```python
from build123d import *

# Parameters (mm, degrees)
SKETCH_1_R          = 15
EXTRUDE_1_DEPTH     = 2
SKETCH_2_R          = 7
EXTRUDE_2_DEPTH     = 10
SKETCH_3_R          = 2
CUT_EXTRUDE_1_DEPTH = 24.452078799
SKETCH_4_R          = 5
CUT_EXTRUDE_2_DEPTH = 25.372115214
CHAMFER_1_SIZE      = 0.2
SKETCH_5_R          = 1.75
CUT_EXTRUDE_3_DEPTH = 10


with BuildPart() as part:
    # 草图1 → 凸台-拉伸1 (new body)
    with BuildSketch(Plane(origin=(0, 0, 0), x_dir=(0, 0, -1), z_dir=(1, 0, 0))):
        Circle(SKETCH_1_R)
    extrude(amount=EXTRUDE_1_DEPTH)

    # 草图2 → 凸台-拉伸2 (add)
    with BuildSketch(Plane(origin=(2, 0, 0), x_dir=(0, 0, -1), z_dir=(1, 0, 0))):
        Circle(SKETCH_2_R)
    extrude(amount=EXTRUDE_2_DEPTH)

    # 草图3 → 切除-拉伸1 (cut, through all)
    with BuildSketch(Plane(origin=(2, 0, 0), x_dir=(0, 0, -1), z_dir=(1, 0, 0))):
        with Locations((0, 11.313708499)):
            Circle(SKETCH_3_R)
        with Locations((8, 8)):
            Circle(SKETCH_3_R)
        with Locations((11.313708499, 0)):
            Circle(SKETCH_3_R)
        with Locations((8, -8)):
            Circle(SKETCH_3_R)
        with Locations((0, -11.313708499)):
            Circle(SKETCH_3_R)
        with Locations((-8, -8)):
            Circle(SKETCH_3_R)
        with Locations((-11.313708499, 0)):
            Circle(SKETCH_3_R)
        with Locations((-8, 8)):
            Circle(SKETCH_3_R)
    extrude(amount=-CUT_EXTRUDE_1_DEPTH, mode=Mode.SUBTRACT)

    # 草图4 → 切除-拉伸2 (cut, through all)
    with BuildSketch(Plane(origin=(12, 0, 0), x_dir=(0, 0, -1), z_dir=(1, 0, 0))):
        Circle(SKETCH_4_R)
    extrude(amount=-CUT_EXTRUDE_2_DEPTH, mode=Mode.SUBTRACT)

    # 倒角1
    chamfer_1_edges = [part.edges().sort_by_distance(p)[0] for p in [
        (0, 0, 15),
        (0, 0, 5),
        (12, 0, 5),
        (2, 0, 15),
        (12, 0, 7),
    ]]
    chamfer(chamfer_1_edges, length=CHAMFER_1_SIZE)

    # 草图5 → 切除-拉伸3 (cut)
    with BuildSketch(Plane(origin=(0, 0, 0), x_dir=(1, 0, 0), z_dir=(0, 1, 0))):
        with Locations(Location((7, 0, 0), (0, 0, 90))):
            Circle(SKETCH_5_R)
    extrude(amount=CUT_EXTRUDE_3_DEPTH, mode=Mode.SUBTRACT)


solid = part.part
```
Model file for the job. Use its own axes, mm. A direction names the side the tool comes from. Coordinates: 2 decimals unless noted, no trailing zeros. Loops run counter-clockwise (first coordinate to the right, second up) from the corner with the lowest first, then second, coordinate; pieces in that order, holes last. Notation, with made-up numbers: (86, 14) -> (101, 14) arc R21 ccw to (101, 31) -> close; hole circle Ø7 at (-4.75, 50.25). An arc over 180 degrees is marked (long way). Answer as a JSON object with one key per item and string values.
Q1. Cut at C-C (x = 10.25). List the corners of the cut face in (y, z).
Report:
{"outline": "circle Ø14 at (0, 0); hole circle Ø10 at (0, 0)"}
Q2. Flat gauge pins, fed straight in: P1, Ø2, axis at x = 8.5, z = -2, coming from the +Y side; P2, Ø3, axis at x = 7, z = 0, coming from the -Y side; P3, Ø6, axis at x = 8.5, y = -1.5, coming from the +Z side; P4, Ø5, axis at x = 6.5, y = -10, coming from the +Z side. Where does each tip first touch, or does it go through?
Report:
{"P1": "stops at y = 6.93", "P2": "stops at y = -7", "P3": "stops at z = 7", "P4": "passes through"}
Q3. Probe probe 1 along Y at (x, z) = (1.05, 0); probe 2 along Y at (x, z) = (0.5, -8); probe 3 along Y at (x, z) = (6.5, 0.25). List the from-to ranges inside material, lowest first.
Report:
{"probe 1": "y = -15 to -13.31, -9.31 to -5, 5 to 9.31, 13.31 to 15", "probe 2": "y = -12.69 to -10, -6 to 6, 10 to 12.69", "probe 3": "y = -7 to -4.99"}
Q4. Cut at A-A (z = 0). State how many separate pieces and enclosed holes the cut face has, and give its area (3 significant figures).
Report:
{"separate pieces": "5", "enclosed holes": "0", "area": "56.8 mm2"}
Q5. Pull direction X, two halves, no side cores. Call faces 3 (the cylindrical face through (6.474, 5.829, -1.669)), 4 (the flat face through (12, -5, 2)), 5 (the cylindrical face through (1.01, 9.36, 0.43)): released by +X, released by -X, zero draft, split by the parting line, or undercut.
Report:
{"face 3": "undercut", "face 4": "released by +X", "face 5": "zero draft"}
Q6. 3-axis set-ups, long thin cutter, end or side, ignore diameter. For faces 1 (the flat face through (0, -6, 0)), 2 (the cylindrical face through (6.831, -6.834, 1.517)): which of +Z, -Z, +X, -X, +Y, -Y reach the whole face in a straight line?
Report:
{"face 1": "+Z, -Z, -X, +Y, -Y", "face 2": "+X"}
